The model under review builds one solid part; all positions refer to its coordinate system, in mm. A direction names the side the tool comes from. Give positions to 0.01 mm unless a question says otherwise; leave off trailing zeros. Order: outer loops, then holes, each group sorted by start corner. A loop starts at its lowest first (then second) coordinate and runs counter-clockwise, first axis right, second up. Notation, with made-up numbers: (80, 36) -> (119, 36) arc R22 cw to (119, 57) -> close; hole circle Ø7 at (69.25, 75). An arc over 180 degrees is marked (long way). Use one line per item in the form item = value.
```python
from build123d import *

# Parameters (mm, degrees)
SKICA1_W                      = 160
SKICA1_H                      = 48
P_IDAT_VYSUNUT_M1_DEPTH       = 3
SKICA3_R                      = 6
SKICA3_R_2                    = 1.375
STOJNY_K_PCB_DEPTH            = 13
SKICA5_W                      = 174
SKICA5_H                      = 62
SKICA5_W_2                    = 160
SKICA5_H_2                    = 48
P_IDAT_VYSUNUT_M3_DEPTH       = 13
ODEBRAT_VYSUNUT_M2_DEPTH      = 177.303715219
ODEBRAT_VYSUNUT_M2_DEPTH_BACK = 177.303715219
SKICA7_R                      = 1.5


with BuildPart() as part:
    # Skica1 → Přidat vysunutím1 (new body)
    with BuildSketch(Plane.XY):
        with Locations((80, 24)):
            Rectangle(SKICA1_W, SKICA1_H)
    extrude(amount=P_IDAT_VYSUNUT_M1_DEPTH)

    # Skica3 → stojny k PCB (add)
    # profile 1 of 4: a face of its own
    with BuildSketch(Plane(origin=(0, 0, 0), x_dir=(-1, 0, 0), z_dir=(0, 0, -1))):
        with Locations((-7.6, 25)):
            Circle(SKICA3_R)
        with Locations((-7.6, 25)):
            Circle(SKICA3_R_2, mode=Mode.SUBTRACT)
    # profile 2 of 4: a face of its own
    with BuildSketch(Plane(origin=(0, 0, 0), x_dir=(-1, 0, 0), z_dir=(0, 0, -1))):
        with Locations((-8.3, 9.7)):
            Circle(SKICA3_R)
        with Locations((-8.3, 9.7)):
            Circle(SKICA3_R_2, mode=Mode.SUBTRACT)
    # profile 3 of 4: a face of its own
    with BuildSketch(Plane(origin=(0, 0, 0), x_dir=(-1, 0, 0), z_dir=(0, 0, -1))):
        with Locations((-142.7, 26.2)):
            Circle(SKICA3_R)
        with Locations((-142.7, 26.2)):
            Circle(SKICA3_R_2, mode=Mode.SUBTRACT)
    # profile 4 of 4: a face of its own
    with BuildSketch(Plane(origin=(0, 0, 0), x_dir=(-1, 0, 0), z_dir=(0, 0, -1))):
        with Locations((-142.7, 8.4)):
            Circle(SKICA3_R)
        with Locations((-142.7, 8.4)):
            Circle(SKICA3_R_2, mode=Mode.SUBTRACT)
    extrude(amount=-STOJNY_K_PCB_DEPTH)

    # Skica5 → Přidat vysunutím3 (add)
    with BuildSketch(Plane(origin=(0, 0, 0), x_dir=(-1, 0, 0), z_dir=(0, 0, -1))):
        with Locations((-80, 24)):
            Rectangle(SKICA5_W, SKICA5_H)
        with Locations((-80, 24)):
            Rectangle(SKICA5_W_2, SKICA5_H_2, mode=Mode.SUBTRACT)
    extrude(amount=-P_IDAT_VYSUNUT_M3_DEPTH)

    # Skica7 → Odebrat vysunutím2 (cut, two sides: drawn at the far end of the back side and taken through both)
    with BuildSketch(Plane.XY.offset(13).offset(-ODEBRAT_VYSUNUT_M2_DEPTH_BACK)):
        with Locations((-3.5, -3.5)):
            Circle(SKICA7_R)
        with Locations((-3.5, 51.5)):
            Circle(SKICA7_R)
        with Locations((163.5, -3.5)):
            Circle(SKICA7_R)
        with Locations((163.5, 51.5)):
            Circle(SKICA7_R)
    extrude(amount=ODEBRAT_VYSUNUT_M2_DEPTH + ODEBRAT_VYSUNUT_M2_DEPTH_BACK, mode=Mode.SUBTRACT)


solid = part.part
```
1. For L1, parallel to X at y = 51.5, z = 9; L2, parallel to Y at x = 52, z = 5; L3, parallel to Y at x = 163.5, z = 5.75, list the stretches that pass through material, from the lowest coordinate up.
Values:
L1 = -7 to -5, -2 to 162, 165 to 167
L2 = -7 to 0, 48 to 55
L3 = -7 to -5, -2 to 50, 53 to 55
2. For pin 1 Ø2.5 at (x, y) = (-3.5, -3.5) entering from -Z; pin 2 Ø0.8 at (x, y) = (8, 25.5) entering from +Z, all flat-tipped, find the tip position at first contact; note any pin that passes through.
Values:
pin_1 = through
pin_2 = 3
3. The part is to be moulded in two halves that separate along X. For faces 3 (the face through (80, 49, 13)), 4 (the face through (-3.825, 50.036, 6.409)), 5 (the face through (-7, 24, 6)), say which applies: +X half, -X half, draft (parallel to the pull), parting line (faces both ways), or undercut.
Values:
face_3 = draft
face_4 = undercut
face_5 = -X half
4. Add section B-B on x = 163.5. Give the boundary of the cut face in (y, z).
Values:
outline = (-7, 0) -> (-5, 0) -> (-5, 13) -> (-7, 13) -> close; (-2, 0) -> (50, 0) -> (50, 13) -> (-2, 13) -> close; (53, 0) -> (55, 0) -> (55, 13) -> (53, 13) -> close
5. Tool access review of faces 1 (the face through (6, 24, 13)), 2 (the face through (0, 24, 8)): name each direction out of +Z, -Z, +X, -X, +Y, -Y from which nothing blocks a thin tool from reaching the whole face with its end or side.
Values:
face_1 = +Z, +X, -X, +Y, -Y
face_2 = +Z
6. Add section D-D on x = 122.5. Give the boundary of the cut face in (y, z), then the cut area to 3 significant figures.
Values:
outline = (-7, 0) -> (55, 0) -> (55, 13) -> (48, 13) -> (48, 3) -> (0, 3) -> (0, 13) -> (-7, 13) -> close
area = 326 mm^2
7. Add section A-A on z = 5.5. Count the separate pieces of the cut face and the enclosed holes in it, then the cut area to 3 significant figures.
Values:
separate_pieces = 5
enclosed_holes = 9
area = 3,510 mm^2
8. Add section C-C on y = 51.5. Give the boundary of the cut face in (x, z), then the cut area to 3 significant figures.
Values:
outline = (-7, 0) -> (-5, 0) -> (-5, 13) -> (-7, 13) -> close; (-2, 0) -> (162, 0) -> (162, 13) -> (-2, 13) -> close; (165, 0) -> (167, 0) -> (167, 13) -> (165, 13) -> close
area = 2,180 mm^2
